Autodesk Inventor part; units mm, degrees
ref_plane "YZ Plane" through (0, 0, 0) normal (1, 0, 0) x (0, 1, 0)
ref_plane "XZ Plane" through (0, 0, 0) normal (0, 1, 0) x (-1, 0, 0)
ref_plane "XY Plane" through (0, 0, 0) normal (0, 0, 1) x (1, 0, 0)
sketch "Sketch1" plane through (0, 0, 0) normal (0, 0, 1) x (1, 0, 0)
  line L0 (0, 0) -> (620, 0)
  line L1 (110, -188) -> (510, -188)
  line L2 (510, -188) -> (510, -55)
  line L3 (510, -55) -> (620, -55)
  line L4 (620, -55) -> (620, 0)
  line L5 (110, -188) -> (110, -55)
  line L6 (0, -55) -> (0, 0)
  line L7 (0, -55) -> (110, -55)
  point P0 (310, -188)
  point P1 (310, 0)
  dimension "d0" = 620
  dimension "d1" = 188
  dimension "d2" = 400
  dimension "d3" = 133
extrude "Extrusion1" add sketch "Sketch1" along normal blind 10
sketch "Sketch2" plane through (0, 0, 10) normal (0, 0, 1) x (1, 0, 0)
  line L0 (620, 0) -> (0, 0)
  line L1 (510, -188) -> (110, -188)
  line L2 (620, 0) -> (310, 0)
  line L3 (310, 0) -> (310, -188)
  line L4 (310, -188) -> (620, -188)
  line L5 (620, -188) -> (620, 0)
extrude "Extrusion2" cut sketch "Sketch2" against normal through all
sketch "Sketch3" plane through (0, 0, 10) normal (0, 0, 1) x (1, 0, 0)
  circle A0 centre (10, -10) radius 2
  line L0 (310, 0) -> (0, 0)
  line L1 (0, 0) -> (0, -55)
  circle A1 centre (155, -10) radius 2
  circle A2 centre (300, -10) radius 2
  line L2 (310, -188) -> (310, 0)
  line L3 (10, -10) -> (300, -10) construction
  circle A3 centre (120, -178) radius 2
  line L4 (110, -55) -> (110, -188)
  line L5 (110, -188) -> (310, -188)
  circle A4 centre (300, -178) radius 2
  dimension "d8" = 4
  dimension "d9" = 10
  dimension "d10" = 10
  dimension "d11" = 4
  dimension "d12" = 4
  dimension "d13" = 10
  dimension "d14" = 4
  dimension "d15" = 10
  dimension "d16" = 10
  dimension "d17" = 4
  dimension "d18" = 10
  dimension "d19" = 10
extrude "Extrusion3" cut sketch "Sketch3" against normal through all
sketch "Sketch4" plane through (0, 0, 0) normal (0, 0, -1) x (-1, 0, 0)
  line L0 (-310, 0) -> (-310, -188)
  line L1 (-310, -32.5) -> (-328, -32.5)
  line L2 (-328, -32.5) -> (-328, -155.5)
  line L3 (-328, -155.5) -> (-310, -155.5)
  line L4 (-310, -155.5) -> (-310, -32.5)
  circle A0 centre (-320, -46.5) radius 2.5
  circle A1 centre (-320, -141.5) radius 2.5
  line L5 (-320, -46.5) -> (-320, -141.5) construction
  point P0 (0, 0)
  point P1 (-310, -94)
  point P2 (-320, -94)
  dimension "d22" = 18
  dimension "d23" = 123
  dimension "d24" = 5
  dimension "d25" = 5
  dimension "d26" = 10
  dimension "d27" = 95
extrude "Extrusion4" add sketch "Sketch4" against normal blind 5
sketch "Sketch6" plane through (0, 0, 10) normal (0, 0, 1) x (1, 0, 0)
  line L0 (286, -59) -> (334, -59)
  line L1 (334, -59) -> (334, -129)
  line L2 (334, -129) -> (286, -129)
  line L3 (286, -129) -> (286, -59)
  line L4 (310, -188) -> (310, 0)
  point P0 (0, 0)
  point P1 (310, -94)
  point P2 (310, -94)
  point P3 (286, -94)
  point P4 (310, -94)
  point P5 (310, -59)
  dimension "d42" = 48
  dimension "d43" = 70
extrude "Extrusion6" add sketch "Sketch6" against normal blind 10
sketch "Sketch7" plane through (0, 0, 10) normal (0, 0, 1) x (1, 0, 0)
  line L0 (324, -69) -> (296, -69)
  line L1 (296, -69) -> (296, -119)
  line L2 (296, -119) -> (324, -119)
  line L3 (324, -119) -> (324, -69)
  line L4 (310, -59) -> (310, 0)
  line L5 (334, -59) -> (334, -129)
  line L6 (290.0321, -94) -> (329.9679, -94) construction
  circle A0 centre (329.9679, -94) radius 1.5
  circle A1 centre (290.0321, -94) radius 1.5
  point P0 (0, 0)
  point P1 (324, -94)
  point P2 (334, -94)
  point P3 (310, -69)
  point P4 (310, -94)
  dimension "d46" = 28
  dimension "d47" = 50
  dimension "d50" = 39.9357
  dimension "d51" = 3
  dimension "d52" = 3
extrude "Extrusion7" cut sketch "Sketch7" against normal through all
properties part number "SP001b" material "ABS Plastic"
The listing builds one solid part. Answer for the finished solid, in the listing's coordinates (mm). A direction names the side the tool comes from. Give positions to 0.01 mm unless a question says otherwise; leave off trailing zeros. Order: outer loops, then holes, each group sorted by start corner. A loop starts at its lowest first (then second) coordinate and runs counter-clockwise, first axis right, second up. Notation, with made-up numbers: (61, 28) - (113, 28) arc R31 ccw to (113, 57) - close; hole circle Ø5 at (-6, 59.25). An arc over 180 degrees is marked (long way). Use one line per item in the form item = value.
1) Each of these flat-tipped pins is pushed along its axis until it touches: pin 1 (6.5 mm diameter, centred on x = 320, y = -46.5, fed in from +Z); pin 2 (3 mm diameter, centred on y = -102.5, z = 4, fed in from -X); pin 3 (5 mm diameter, centred on x = 66, z = 3.5, fed in from -Y). Where does it stop, or does it pass through?
Verdict:
pin_1 = 5
pin_2 = 110
pin_3 = -55
2) The mould has two halves that part along Y. Classify faces 5 (the flat face through (310, -69, 5)), 6 (the flat face through (296, -94, 5)), 7 (the flat face through (209, -188, 5)), 8 (the flat face through (0, -28, 5)): released by +Y, released by -Y, zero draft, split by the parting line, or undercut.
Verdict:
face_5 = undercut
face_6 = undercut
face_7 = released by -Y
face_8 = zero draft
3) Find section C-C on x = 95. Determine the outline of the cut face in (y, z), and give its area (3 significant figures).
Verdict:
outline = (-55, 0) - (0, 0) - (0, 10) - (-55, 10) - close
area = 550 mm^2
4) Find section D-D on y = -152. Determine the outline of the cut face in (x, z).
Verdict:
outline = (110, 0) - (328, 0) - (328, 5) - (310, 5) - (310, 10) - (110, 10) - close
5) Find section B-B on y = -101.5. Determine the outline of the cut face in (x, z), and give its area (3 significant figures).
Verdict:
outline = (110, 0) - (296, 0) - (296, 10) - (110, 10) - close; (324, 0) - (334, 0) - (334, 10) - (324, 10) - close
area = 1,960 mm^2
6) Consider probe 1 along X at (y, z) = (-94, 2); probe 2 along Y at (x, z) = (320, 2.7); probe 3 along Y at (x, z) = (300, 4). Determine where each line is inside the solid, lowest interval first. Write a range as [from, to].
Verdict:
probe_1 = [110, 288.53], [291.53, 296], [324, 328.47], [331.47, 334]
probe_2 = [-155.5, -144], [-139, -119], [-69, -49], [-44, -32.5]
probe_3 = [-188, -180], [-176, -119], [-69, -12], [-8, 0]
7) Find section A-A on z = 3. Give the number of separate pieces and of enclosed holes in the cut face, and give its area (3 significant figures).
Verdict:
separate_pieces = 1
enclosed_holes = 10
area = 44,800 mm^2
8) For faces 1 (the flat face through (317, -46, 5)), 2 (the flat face through (317, -142, 5)), 3 (the flat face through (110, -122, 5)), 4 (the flat face through (324, -94, 5)), determine the directions among +Z, -Z, +X, -X, +Y, -Y from which every point of the face is accessible in a straight line to the end or side of a thin tool.
Verdict:
face_1 = +Z, +X, +Y
face_2 = +Z, +X, -Y
face_3 = +Z, -Z, -X, -Y
face_4 = +Z, -Z
